from build123d import *

# Parameters (mm, degrees)
SKETCH1_W               = 60
SKETCH1_H               = 53.4
SKETCH1_R               = 5
SKETCH1_R_2             = 18
BOSS_EXTRUDE1_DEPTH     = 5
SKETCH1_3_R             = 18
SKETCH1_3_R_2           = 16.5
BOSS_EXTRUDE2_DEPTH     = 30
SKETCH1_4_R             = 16.5
SKETCH1_4_R_2           = 2.5
BOSS_EXTRUDE3_DEPTH     = 10
CUT_EXTRUDE1_DEPTH      = 51.128734275
CUT_EXTRUDE1_DEPTH_BACK = 51.128734275
SKETCH2_R               = 5


with BuildPart() as part:
    # Sketch1 → Boss-Extrude1 (new body)
    with BuildSketch(Plane.XY):
        Rectangle(SKETCH1_W, SKETCH1_H)
        with Locations((-20, -16.7)):
            Circle(SKETCH1_R, mode=Mode.SUBTRACT)
        with Locations((20, -16.7)):
            Circle(SKETCH1_R, mode=Mode.SUBTRACT)
        with Locations((20, 16.7)):
            Circle(SKETCH1_R, mode=Mode.SUBTRACT)
        with Locations((-20, 16.7)):
            Circle(SKETCH1_R, mode=Mode.SUBTRACT)
        Circle(SKETCH1_R_2, mode=Mode.SUBTRACT)
    extrude(amount=BOSS_EXTRUDE1_DEPTH)

    # Sketch1<3> → Boss-Extrude2 (add)
    with BuildSketch(Plane.XY):
        Circle(SKETCH1_3_R)
        Circle(SKETCH1_3_R_2, mode=Mode.SUBTRACT)
    extrude(amount=BOSS_EXTRUDE2_DEPTH)

    # Sketch1<4> → Boss-Extrude3 (add)
    with BuildSketch(Plane.XY):
        Circle(SKETCH1_4_R)
        with Locations((7.5, 0)):
            Circle(SKETCH1_4_R_2, mode=Mode.SUBTRACT)
        with Locations((-7.5, 0)):
            Circle(SKETCH1_4_R_2, mode=Mode.SUBTRACT)
    extrude(amount=BOSS_EXTRUDE3_DEPTH)

    # Sketch2 → Cut-Extrude1 (cut, two sides: drawn at the far end of the back side and taken through both)
    with BuildSketch(Plane(origin=(0, 0, 0), x_dir=(0, 0, -1), z_dir=(1, 0, 0)).offset(-CUT_EXTRUDE1_DEPTH_BACK)):
        with Locations((-16.460509222, 0.48266687)):
            Circle(SKETCH2_R)
    extrude(amount=CUT_EXTRUDE1_DEPTH + CUT_EXTRUDE1_DEPTH_BACK, mode=Mode.SUBTRACT)


solid = part.part
Design review of the part built by this model. Coordinates are the model's own, in mm. A direction names the side the tool comes from. Coordinates: 2 decimals unless noted, no trailing zeros. Order: outer loops, then holes, each group sorted by start corner. A loop starts at its lowest first (then second) coordinate and runs counter-clockwise, first axis right, second up. Notation, with made-up numbers: M 43,60 L 67,60 A20 ccw 67,76 Z; hole C 29.25,59.5 d3. An arc over 180 degrees is marked long. Use a Markdown table: item, result.
(1) Add section B-B (z = 4). Give the boundary of the cut face in (x, y).
Worked answers:
| item | result |
|---|---|
| outline | M -30,-26.7 L 30,-26.7 L 30,26.7 L -30,26.7 Z; hole C -20,-16.7 d10; hole C -20,16.7 d10; hole C -7.5,0 d5; hole C 7.5,0 d5; hole C 20,-16.7 d10; hole C 20,16.7 d10 |
(2) For P1, Ø10, axis at x = -4, y = 5, coming from the +Z side; P2, Ø1, axis at x = -4.5, y = -21, coming from the +Z side; P3, Ø10, axis at y = 13, z = 24.5, coming from the +X side, all flat-tipped, find the tip position at first contact; note any pin that passes through.
Worked answers:
| item | result |
|---|---|
| P1 | stops at z = 10 |
| P2 | stops at z = 5 |
| P3 | stops at x = 16.12 |
(3) Wall thickness on probe 1 along Y at (x, z) = (-20, 3); probe 2 along Z at (x, y) = (4, -3.5); probe 3 along X at (y, z) = (-2, 25): over which ranges is each line inside the solid? List them lowest first.
Worked answers:
| item | result |
|---|---|
| probe 1 | y = -26.7 to -21.7, -11.7 to 11.7, 21.7 to 26.7 |
| probe 2 | z = 0 to 10 |
| probe 3 | x = -17.89 to -16.38, 16.38 to 17.89 |
(4) Add section C-C (y = 14.5). Give the boundary of the cut face in (x, z), then the cut area to 3 significant figures.
Worked answers:
| item | result |
|---|---|
| outline | M -30,0 L -24.49,0 L -24.49,5 L -30,5 Z; M -15.51,0 L 15.51,0 L 15.51,5 L 10.67,5 L 10.67,30 L 7.87,30 L 7.87,10 L -7.87,10 L -7.87,30 L -10.67,30 L -10.67,5 L -15.51,5 Z; M 24.49,0 L 30,0 L 30,5 L 24.49,5 Z |
| area | 429 mm2 |
(5) For faces 1 (the cylindrical face through (-10, 0, 5)), 2 (the cylindrical face through (16.63, -6.89, 17.32)), list the 3-axis set-ups (+Z, -Z, +X, -X, +Y, -Y) from which the entire face can be reached by the end or side of a thin tool; tool diameter is ignored.
Worked answers:
| item | result |
|---|---|
| face 1 | +Z, -Z |
| face 2 | +Z |
(6) Draft analysis for pull direction Y (two halves, no side actions). For faces 3 (the flat face through (0, 0, 10)), 4 (the flat face through (30, 0, 2)), 5 (the flat face through (0, -26.7, 2)), state which applies: released by +Y, released by -Y, zero draft, split by the parting line, or undercut.
Worked answers:
| item | result |
|---|---|
| face 3 | undercut |
| face 4 | zero draft |
| face 5 | released by -Y |
(7) Add section D-D (x = -7.5). Give the boundary of the cut face in (y, z).
Worked answers:
| item | result |
|---|---|
| outline | M -26.7,0 L -2.5,0 L -2.5,10 L -14.7,10 L -14.7,30 L -16.36,30 L -16.36,5 L -26.7,5 Z; M 2.5,0 L 26.7,0 L 26.7,5 L 16.36,5 L 16.36,30 L 14.7,30 L 14.7,10 L 2.5,10 Z |
(8) Add section A-A (x = 20). Give the boundary of the cut face in (y, z), then the cut area to 3 significant figures.
Worked answers:
| item | result |
|---|---|
| outline | M -26.7,0 L -21.7,0 L -21.7,5 L -26.7,5 Z; M -11.7,0 L 11.7,0 L 11.7,5 L -11.7,5 Z; M 21.7,0 L 26.7,0 L 26.7,5 L 21.7,5 Z |
| area | 167 mm2 |
